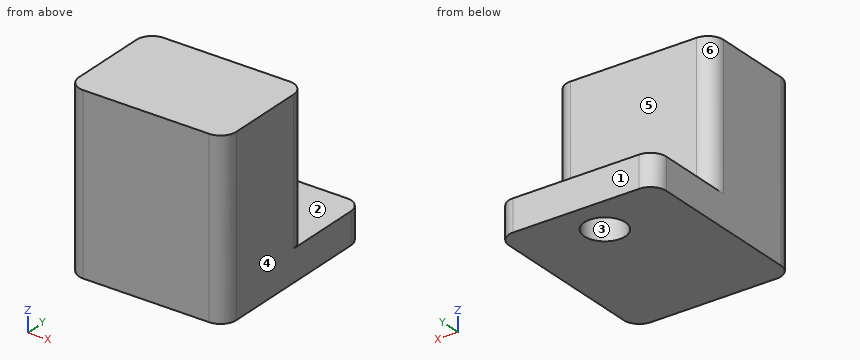
from build123d import *

# Parameters (mm, degrees)
SKETCH001_W  = 10
SKETCH001_H  = 7
PAD001_DEPTH = 9
SKETCH_W     = 10
SKETCH_H     = 12
SKETCH_R     = 1.3
PAD_DEPTH    = 2
FILLET_R     = 1
FILLET001_R  = 1


with BuildPart() as pad001:
    # Sketch001 → Pad001 (new body)
    with BuildSketch(Plane.XY):
        with Locations((0, 3.5)):
            Rectangle(SKETCH001_W, SKETCH001_H)
    extrude(amount=PAD001_DEPTH)


with BuildPart() as fillet001:
    # Sketch → Pad (new body)
    with BuildSketch(Plane.XY):
        with Locations((0, 6)):
            Rectangle(SKETCH_W, SKETCH_H)
        with Locations((0, 9.5)):
            Circle(SKETCH_R, mode=Mode.SUBTRACT)
    extrude(amount=-PAD_DEPTH)

    # Fusion: union Pad001
    add(pad001.part)

    # Fillet
    fillet_edges = [fillet001.edges().sort_by_distance(p)[0] for p in [
        (5, 0, 4.5),
        (5, 0, -1),
    ]]
    fillet(fillet_edges, radius=FILLET_R)

    # Fillet001
    fillet001_edges = [fillet001.edges().sort_by_distance(p)[0] for p in [
        (-5, 0, 4.5),
        (-5, 0, -1),
        (-5, 7, 4.5),
        (-5, 12, -1),
        (5, 7, 4.5),
        (5, 12, -1),
    ]]
    fillet(fillet001_edges, radius=FILLET001_R)


solid = fillet001.part
Can you work these out from the model? Positions are in its coordinate system, mm. Face numbers are marked on the shaded views. A direction names the side the tool comes from. Round coordinates to 2 decimals unless told otherwise and drop trailing zeros. Write each loop counter-clockwise with the first axis right and the second up, starting at its lowest first coordinate (ties: lowest second). Pieces come first, ordered by that corner, then holes. Notation, with made-up numbers: (78, -32.5) -> (84, -32.5) arc R28 ccw to (84, -10.5) -> close; hole circle Ø4 at (72.25, 45). An arc over 180 degrees is marked (long way). One line per question, with ' | ' between items. Start each with the question number.
1) On a 3-axis mill with a long thin cutter (end or side, diameter ignored), from which of +Z, -Z, +X, -X, +Y, -Y can I reach the whole of each face in a straight line? I mean the marked faces 4, 5 and 6. Say none if no direction works.
2) If we mould it in two halves opening along Y, with no side actions, what happens to the marked faces 1, 2 and 3? For each: released by +Y, released by -Y, zero draft, split by the parting line, or undercut.
3) I'm going to push a flat-ended pin straight in: P1, Ø4, axis at x = 0, y = 9.5, coming from the +Z side. Where does the tip first touch, or does it pass through?
4) Suppose I cut it at D-D on z = 5.75. Write out the boundary of the cut face in (x, y), then the cut area to 3 significant figures.
5) Suppose I cut it at A-A on x = 0. Write out the boundary of the cut face in (y, z).
6) Suppose I cut it at C-C on z = -1. Write out the boundary of the cut face in (x, y).
7) Suppose I cut it at B-B on y = 9.5. Write out the boundary of the cut face in (x, z), then the cut area to 3 significant figures.
8) I need wall thicknesses on line 1 (Y direction, x = 0, z = -1.45); line 2 (Y direction, x = 3, z = 6.25); line 3 (Z direction, x = -1.5, y = 8). Which ranges of each line are inside material? Lowest first, please. Write a range as [from, to].
Return value:
1) face 4: +Z, -Z, +X, +Y, -Y | face 5: +Z, +X, -X, +Y | face 6: +Z, -X, +Y
2) face 1: released by +Y | face 2: zero draft | face 3: undercut
3) P1: stops at z = 0
4) outline: (-5, 1) arc R1 ccw to (-4, 0) -> (4, 0) arc R1 ccw to (5, 1) -> (5, 6) arc R1 ccw to (4, 7) -> (-4, 7) arc R1 ccw to (-5, 6) -> close | area: 69.1 mm2
5) outline: (0, -2) -> (8.2, -2) -> (8.2, 0) -> (7, 0) -> (7, 9) -> (0, 9) -> close; (10.8, -2) -> (12, -2) -> (12, 0) -> (10.8, 0) -> close
6) outline: (-5, 1) arc R1 ccw to (-4, 0) -> (4, 0) arc R1 ccw to (5, 1) -> (5, 11) arc R1 ccw to (4, 12) -> (-4, 12) arc R1 ccw to (-5, 11) -> close; hole circle Ø2.6 at (0, 9.5)
7) outline: (-5, -2) -> (-1.3, -2) -> (-1.3, 0) -> (-5, 0) -> close; (1.3, -2) -> (5, -2) -> (5, 0) -> (1.3, 0) -> close | area: 14.8 mm2
8) line 1: y = [0, 8.2], [10.8, 12] | line 2: y = [0, 7] | line 3: z = [-2, 0]
